```python
from build123d import *

# Parameters (mm, degrees)
SKETCH3_W           = 70
SKETCH3_H           = 60
BOSS_EXTRUDE3_DEPTH = 20
SKETCH4_R           = 1.65
CUT_EXTRUDE1_DEPTH  = 95.339811321
SKETCH6_R           = 2.1
CUT_EXTRUDE2_DEPTH  = 95.339811321
SKETCH9_R           = 3.375
CUT_EXTRUDE3_DEPTH  = 40.25
CUT_EXTRUDE4_START  = -3
SKETCH11_R          = 3
SKETCH11_R_2        = 1.65
CUT_EXTRUDE4_DEPTH  = 3
CUT_EXTRUDE5_DEPTH  = 5
CHAMFER2_SIZE       = 0.8


with BuildPart() as part:
    # Sketch3 → Boss-Extrude3 (new body)
    with BuildSketch(Plane(origin=(0, 0, 0), x_dir=(1, 0, 0), z_dir=(0, 1, 0))):
        with Locations((35, -30)):
            Rectangle(SKETCH3_W, SKETCH3_H)
    extrude(amount=BOSS_EXTRUDE3_DEPTH)

    # Sketch4 → Cut-Extrude1 (cut, through all)
    with BuildSketch(Plane(origin=(0, 20, 0), x_dir=(1, 0, 0), z_dir=(0, 1, 0))):
        with Locations(Location((35, -30, 0), (0, 0, 270))):
            Circle(SKETCH4_R)
        with Locations(Location((35, -18, 0), (0, 0, 270))):
            Circle(SKETCH4_R)
        with Locations(Location((47, -30, 0), (0, 0, 270))):
            Circle(SKETCH4_R)
        with Locations(Location((35, -42, 0), (0, 0, 270))):
            Circle(SKETCH4_R)
        with Locations(Location((23, -30, 0), (0, 0, 270))):
            Circle(SKETCH4_R)
    extrude(amount=-CUT_EXTRUDE1_DEPTH, mode=Mode.SUBTRACT)

    # Sketch6 → Cut-Extrude2 (cut, through all)
    with BuildSketch(Plane.XZ):
        with Locations(Location((25.625, 38.125, 0), (0, 0, 270))):
            Circle(SKETCH6_R)
        with Locations(Location((59.875, 38.125, 0), (0, 0, 270))):
            Circle(SKETCH6_R)
    extrude(amount=-CUT_EXTRUDE2_DEPTH, mode=Mode.SUBTRACT)

    # Sketch9 → Cut-Extrude3 (cut)
    with BuildSketch(Plane(origin=(0, 0, 60), x_dir=(-1, 0, 0), z_dir=(0, 0, -1))):
        with Locations((-52.4, 7.5)):
            Circle(SKETCH9_R)
        with Locations((-15.975, 7.5)):
            Circle(SKETCH9_R)
    extrude(amount=CUT_EXTRUDE3_DEPTH, mode=Mode.SUBTRACT)

    # Sketch11 → Cut-Extrude4 (cut)
    # profile 1 of 10: a face of its own
    with BuildSketch(Plane.XZ.offset(CUT_EXTRUDE4_START)):
        with Locations(Location((35, 18, 0), (0, 0, 270))):
            Circle(SKETCH11_R)
        with Locations(Location((35, 18, 0), (0, 0, 90))):
            Circle(SKETCH11_R_2, mode=Mode.SUBTRACT)
    # profile 2 of 10: a face of its own
    with BuildSketch(Plane.XZ.offset(CUT_EXTRUDE4_START)):
        with Locations(Location((35, 30, 0), (0, 0, 270))):
            Circle(SKETCH11_R)
        with Locations(Location((35, 30, 0), (0, 0, 90))):
            Circle(SKETCH11_R_2, mode=Mode.SUBTRACT)
    # profile 3 of 10: a face of its own
    with BuildSketch(Plane.XZ.offset(CUT_EXTRUDE4_START)):
        with Locations(Location((47, 30, 0), (0, 0, 270))):
            Circle(SKETCH11_R)
        with Locations(Location((47, 30, 0), (0, 0, 90))):
            Circle(SKETCH11_R_2, mode=Mode.SUBTRACT)
    # profile 4 of 10: a face of its own
    with BuildSketch(Plane.XZ.offset(CUT_EXTRUDE4_START)):
        with Locations(Location((23, 30, 0), (0, 0, 270))):
            Circle(SKETCH11_R)
        with Locations(Location((23, 30, 0), (0, 0, 90))):
            Circle(SKETCH11_R_2, mode=Mode.SUBTRACT)
    # profile 5 of 10: a face of its own
    with BuildSketch(Plane.XZ.offset(CUT_EXTRUDE4_START)):
        with Locations(Location((35, 42, 0), (0, 0, 270))):
            Circle(SKETCH11_R)
        with Locations(Location((35, 42, 0), (0, 0, 90))):
            Circle(SKETCH11_R_2, mode=Mode.SUBTRACT)
    # profile 6 of 10: a face of its own
    with BuildSketch(Plane.XZ.offset(CUT_EXTRUDE4_START)):
        with Locations(Location((35, 42, 0), (0, 0, 90))):
            Circle(SKETCH11_R_2)
    # profile 7 of 10: a face of its own
    with BuildSketch(Plane.XZ.offset(CUT_EXTRUDE4_START)):
        with Locations(Location((23, 30, 0), (0, 0, 90))):
            Circle(SKETCH11_R_2)
    # profile 8 of 10: a face of its own
    with BuildSketch(Plane.XZ.offset(CUT_EXTRUDE4_START)):
        with Locations(Location((35, 30, 0), (0, 0, 90))):
            Circle(SKETCH11_R_2)
    # profile 9 of 10: a face of its own
    with BuildSketch(Plane.XZ.offset(CUT_EXTRUDE4_START)):
        with Locations(Location((47, 30, 0), (0, 0, 90))):
            Circle(SKETCH11_R_2)
    # profile 10 of 10: a face of its own
    with BuildSketch(Plane.XZ.offset(CUT_EXTRUDE4_START)):
        with Locations(Location((35, 18, 0), (0, 0, 90))):
            Circle(SKETCH11_R_2)
    extrude(amount=CUT_EXTRUDE4_DEPTH, mode=Mode.SUBTRACT)

    # Sketch12 → Cut-Extrude5 (cut)
    with BuildSketch(Plane(origin=(0, 20, 0), x_dir=(1, 0, 0), z_dir=(0, 1, 0))):
        with BuildLine():
            Line((9.45, -60.104949747), (9.45, -44.5))
            ThreePointArc((9.45, -44.5), (14.5, -39.45), (19.55, -44.5))
            Line((19.55, -44.5), (19.55, -60.104949747))
            ThreePointArc((19.55, -60.104949747), (14.5, -65.154949747), (9.45, -60.104949747))
        make_face()
        with BuildLine():
            Line((60.55, -60.104949747), (60.55, -44.5))
            ThreePointArc((60.55, -44.5), (55.5, -39.45), (50.45, -44.5))
            Line((50.45, -44.5), (50.45, -60.104949747))
            ThreePointArc((50.45, -60.104949747), (55.5, -65.154949747), (60.55, -60.104949747))
        make_face()
        with BuildLine():
            Line((60.55, 0.104949747), (60.55, -15.5))
            ThreePointArc((60.55, -15.5), (55.5, -20.55), (50.45, -15.5))
            Line((50.45, -15.5), (50.45, 0.104949747))
            ThreePointArc((50.45, 0.104949747), (55.5, 5.154949747), (60.55, 0.104949747))
        make_face()
        with BuildLine():
            Line((9.45, 0.104949747), (9.45, -15.5))
            ThreePointArc((9.45, -15.5), (14.5, -20.55), (19.55, -15.5))
            Line((19.55, -15.5), (19.55, 0.104949747))
            ThreePointArc((19.55, 0.104949747), (14.5, 5.154949747), (9.45, 0.104949747))
        make_face()
    extrude(amount=-CUT_EXTRUDE5_DEPTH, mode=Mode.SUBTRACT)

    # Chamfer2
    chamfer2_edges = [part.edges().sort_by_distance(p)[0] for p in [
        (55.775, 7.5, 60),
        (19.35, 7.5, 60),
    ]]
    chamfer(chamfer2_edges, length=CHAMFER2_SIZE)


solid = part.part
```
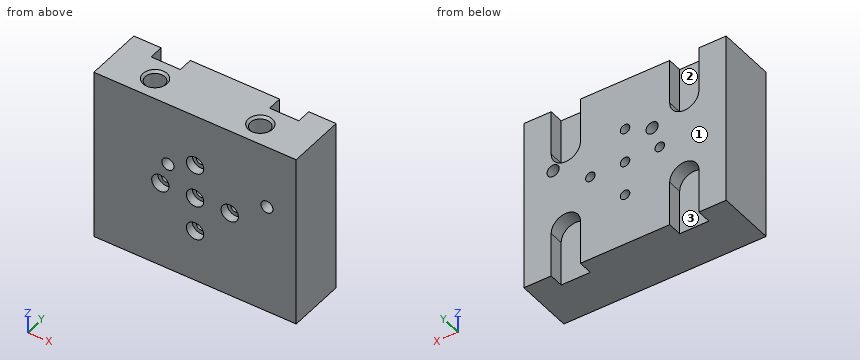
Part model, mm, in its own coordinate system. Face numbers are marked on the shaded views. A direction names the side the tool comes from. Coordinates: 2 decimals unless noted, no trailing zeros. Loops run counter-clockwise (first coordinate to the right, second up) from the corner with the lowest first, then second, coordinate; pieces in that order, holes last. Notation, with made-up numbers: (-4, 73) - (40, 73) arc R17 cw to (40, 100) - close; hole circle Ø1 at (24.5, -9). An arc over 180 degrees is marked (long way). Write item = value, one per line. Start each with the question number.
Item 1: Flat gauge pins, fed straight in: pin 1 Ø3 at (x, z) = (55, 45) entering from +Y; pin 2 Ø3 at (x, z) = (35, 42) entering from -Y; pin 3 Ø4 at (x, z) = (23, 30) entering from -Y; pin 4 Ø8 at (x, y) = (52.4, 7.5) entering from +Z (3 decimals). Where does each tip first touch, or does it go through?
Item 2: Cut at D-D, the plane z = 18. Give the cut face in (x, y), and give its area (3 significant figures).
Item 3: Cut at B-B, the plane z = 48.5. Give the cut face in (x, y) (3 decimals), and give its area (3 significant figures).
Item 4: Cut at C-C, the plane y = 17.75. Give the cut face in (x, z) (3 decimals).
Item 5: Cut at A-A, the plane x = 35. Give the cut face in (y, z).
Item 6: Wall check: L1, parallel to X at y = 1.85, z = 30; L2, parallel to Z at x = 33.5, y = 17.5; L3, parallel to X at y = 5.5, z = 31.5. Give the ranges that are in metal, low to high. Write a range as from..to.
Item 7: 3-axis set-ups, long thin cutter, end or side, ignore diameter. For the marked faces 1, 2 and 3: which of +Z, -Z, +X, -X, +Y, -Y reach the whole face in a straight line?
The answers:
q1.pin_1 = 15
q1.pin_2 = through
q1.pin_3 = 3
q1.pin_4 = 59.825
q2.outline = (0, 0) - (32, 0) - (32, 3) - (33.35, 3) - (33.35, 20) - (18.89, 20) - (18.89, 15) - (10.11, 15) - (10.11, 20) - (0, 20) - close; (36.65, 3) - (38, 3) - (38, 0) - (70, 0) - (70, 20) - (59.89, 20) - (59.89, 15) - (51.11, 15) - (51.11, 20) - (36.65, 20) - close
q2.area = 1,240 mm2
q3.outline = (0, 0) - (70, 0) - (70, 20) - (60.55, 20) - (60.55, 15) - (50.45, 15) - (50.45, 20) - (19.55, 20) - (19.55, 15) - (9.45, 15) - (9.45, 20) - (0, 20) - close; hole circle Ø6.75 at (15.975, 7.5); hole circle Ø6.75 at (52.4, 7.5)
q3.area = 1,230 mm2
q4.outline = (0, 0) - (9.45, 0) - (9.45, 15.5) arc R5.05 cw to (19.55, 15.5) - (19.55, 0) - (50.45, 0) - (50.45, 15.5) arc R5.05 cw to (60.55, 15.5) - (60.55, 0) - (70, 0) - (70, 60) - (60.55, 60) - (60.55, 44.5) arc R5.05 cw to (50.45, 44.5) - (50.45, 60) - (19.55, 60) - (19.55, 44.5) arc R5.05 cw to (9.45, 44.5) - (9.45, 60) - (0, 60) - close; hole circle Ø3.3 at (23, 30); hole circle Ø4.2 at (25.625, 38.125); hole circle Ø3.3 at (35, 18); hole circle Ø3.3 at (35, 30); hole circle Ø3.3 at (35, 42); hole circle Ø3.3 at (47, 30); hole circle Ø4.2 at (59.875, 38.125)
q5.outline = (0, 0) - (20, 0) - (20, 16.35) - (3, 16.35) - (3, 15) - (0, 15) - close; (0, 21) - (3, 21) - (3, 19.65) - (20, 19.65) - (20, 28.35) - (3, 28.35) - (3, 27) - (0, 27) - close; (0, 33) - (3, 33) - (3, 31.65) - (20, 31.65) - (20, 40.35) - (3, 40.35) - (3, 39) - (0, 39) - close; (0, 45) - (3, 45) - (3, 43.65) - (20, 43.65) - (20, 60) - (0, 60) - close
q6.L1 = 0..20, 26..32, 38..44, 50..70
q6.L2 = 0..17.31, 18.69..29.31, 30.69..41.31, 42.69..60
q6.L3 = 0..13.26, 18.69..22.31, 23.69..34.31, 35.69..46.31, 47.69..49.68, 55.12..70
q7.face_1 = +Z, -Z, +X, -X, +Y
q7.face_2 = +Z, +Y
q7.face_3 = -Z, +Y
